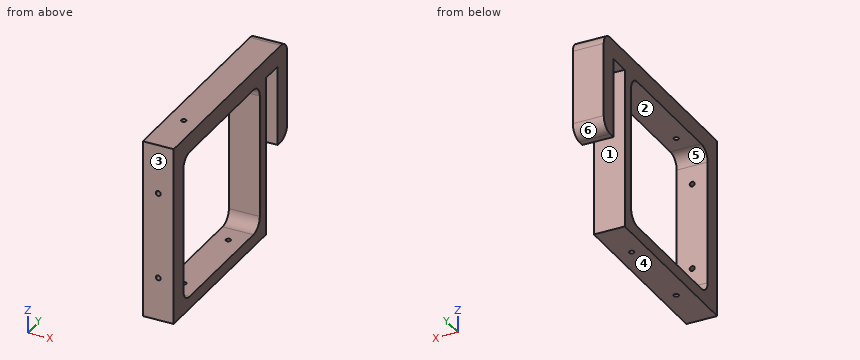
from build123d import *

# Parameters (mm, degrees)
ESQUISSE1_W             = 120
ESQUISSE1_H             = 120
BOSS_EXTRU_1_DEPTH      = 25
ESQUISSE2_R             = 2
ENL_V_MAT_EXTRU_1_DEPTH = 220.588251052
ESQUISSE3_R             = 2
ENL_V_MAT_EXTRU_2_DEPTH = 225.797686821
ESQUISSE4_R             = 2
ENL_V_MAT_EXTRU_3_DEPTH = 222.831016767
CONG_1_R                = 10
CONG_2_R                = 10


with BuildPart() as part:
    # Esquisse1 → Boss.-Extru.1 (new body)
    with BuildSketch(Plane(origin=(0, 0, 0), x_dir=(0, 0, -1), z_dir=(1, 0, 0))):
        Polygon((0, 0), (145, 0), (145, 145), (15, 145), (15, 163), (80, 163), (80, 178), (0, 178), align=None)
        with Locations((75, 75)):
            Rectangle(ESQUISSE1_W, ESQUISSE1_H, mode=Mode.SUBTRACT)
    extrude(amount=BOSS_EXTRU_1_DEPTH)

    # Esquisse2 → Enlèv. mat.-Extru.1 (cut, through all)
    with BuildSketch(Plane(origin=(0, 15, 0), x_dir=(1, 0, 0), z_dir=(0, 1, 0))):
        with Locations(Location((12.5, 40, 0), (0, 0, 270))):
            Circle(ESQUISSE2_R)
        with Locations(Location((12.5, 110, 0), (0, 0, 270))):
            Circle(ESQUISSE2_R)
    extrude(amount=-ENL_V_MAT_EXTRU_1_DEPTH, mode=Mode.SUBTRACT)

    # Esquisse3 → Enlèv. mat.-Extru.2 (cut, through all)
    with BuildSketch(Plane.XY.offset(-135)):
        with Locations((12.5, 40)):
            Circle(ESQUISSE3_R)
        with Locations((12.5, 110)):
            Circle(ESQUISSE3_R)
    extrude(amount=-ENL_V_MAT_EXTRU_2_DEPTH, mode=Mode.SUBTRACT)

    # Esquisse4 → Enlèv. mat.-Extru.3 (cut, through all)
    with BuildSketch(Plane(origin=(0, 0, -15), x_dir=(-1, 0, 0), z_dir=(0, 0, -1))):
        with Locations(Location((-12.5, 40, 0), (0, 0, 180))):
            Circle(ESQUISSE4_R)
    extrude(amount=-ENL_V_MAT_EXTRU_3_DEPTH, mode=Mode.SUBTRACT)

    # Congé1
    cong_1_edges = [part.edges().sort_by_distance(p)[0] for p in [
        (12.5, 178, 0),
        (12.5, 178, -80),
    ]]
    fillet(cong_1_edges, radius=CONG_1_R)

    # Congé2
    cong_2_edges = [part.edges().sort_by_distance(p)[0] for p in [
        (12.5, 135, -135),
        (12.5, 135, -15),
        (12.5, 15, -15),
        (12.5, 15, -135),
    ]]
    fillet(cong_2_edges, radius=CONG_2_R)


solid = part.part
Check sheet for the modelled part. Datum: model origin and axes. Units: mm. Face numbers are marked on the shaded views. A direction names the side the tool comes from. Coordinates: 2 decimals unless noted, no trailing zeros. Write each loop counter-clockwise with the first axis right and the second up, starting at its lowest first coordinate (ties: lowest second). Pieces come first, ordered by that corner, then holes. Notation, with made-up numbers: M -0.75,8.25 L 5.25,8.25 A15 cw 5.25,23.25 Z; hole C 56,53.5 d7. An arc over 180 degrees is marked long. Answer as CSV lines item,"result".
Q1. Mould release check, pull along Y, two halves, no side actions. Record for the marked faces 4, 5 and 6: released by +Y, released by -Y, zero draft, split by the parting line, or undercut.
Check result:
face 4,"zero draft"
face 5,"undercut"
face 6,"released by +Y"
Q2. Material ranges on probe 1 along Y at (x, z) = (12.5, -140.5); probe 2 along Y at (x, z) = (1.75, -28); probe 3 along Y at (x, z) = (18, -82), recorded low to high. Write a range as from..to.
Check result:
probe 1,"0..38, 42..108, 112..145"
probe 2,"0..15, 135..145, 163..178"
probe 3,"0..15, 135..145"
Q3. Cross-section at A-A (y = 40). Record the boundary of the cut face in (x, z), then the cut area to 3 significant figures.
Check result:
outline,"M 0,-145 L 10.5,-145 L 10.5,-135 L 0,-135 Z; M 0,-15 L 10.5,-15 L 10.5,0 L 0,0 Z; M 14.5,-145 L 25,-145 L 25,-135 L 14.5,-135 Z; M 14.5,-15 L 25,-15 L 25,0 L 14.5,0 Z"
area,"525 mm^2"
Q4. Set-up check for the marked faces 1, 2 and 3: record each of +Z, -Z, +X, -X, +Y, -Y from which the full face is reachable in a straight line by a thin tool's end or side.
Check result:
face 1,"-Z, +X, -X"
face 2,"+X, -X"
face 3,"+Z, -Z, +X, -X, -Y"
Q5. Cross-section at B-B (z = -40). Record the boundary of the cut face in (x, y), then the cut area to 3 significant figures.
Check result:
outline,"M 0,0 L 10.5,0 L 10.5,15 L 0,15 Z; M 0,135 L 25,135 L 25,145 L 0,145 Z; M 0,163 L 25,163 L 25,178 L 0,178 Z; M 14.5,0 L 25,0 L 25,15 L 14.5,15 Z"
area,"940 mm^2"
Q6. Go/stop test with flat-tipped pins: pin 1 (9 mm diameter, centred on x = 18, y = 154.5, fed in from -Z); pin 2 (3 mm diameter, centred on x = 7, z = -127, fed in from +Y); pin 3 (4 mm diameter, centred on x = 11, y = 165.5, fed in from -Z). Record where each tip stops, or that it passes through.
Check result:
pin 1,"z = -15"
pin 2,"y = 145"
pin 3,"z = -80"
Q7. Cross-section at C-C (y = 110). Record the boundary of the cut face in (x, z), then the cut area to 3 significant figures.
Check result:
outline,"M 0,-145 L 10.5,-145 L 10.5,-135 L 0,-135 Z; M 0,-15 L 25,-15 L 25,0 L 0,0 Z; M 14.5,-145 L 25,-145 L 25,-135 L 14.5,-135 Z"
area,"585 mm^2"
Q8. Cross-section at D-D (z = -110). Record the boundary of the cut face in (x, y), then the cut area to 3 significant figures.
Check result:
outline,"M 0,0 L 10.5,0 L 10.5,15 L 0,15 Z; M 0,135 L 25,135 L 25,145 L 0,145 Z; M 14.5,0 L 25,0 L 25,15 L 14.5,15 Z"
area,"565 mm^2"
